Part print with two shaded views. Sizes in mm from the minimum x, y, z corner. A direction names the side the tool comes from. Round coordinates to 2 decimals unless told otherwise and drop trailing zeros. Order: outer loops, then holes, each group sorted by start corner. A loop starts at its lowest first (then second) coordinate and runs counter-clockwise, first axis right, second up. Notation, with made-up numbers: M 0,35 L 41,35 A28 ccw 41,71 Z; hole C -39,71.25 d11. An arc over 180 degrees is marked long. Put each result on its own line as item: value.
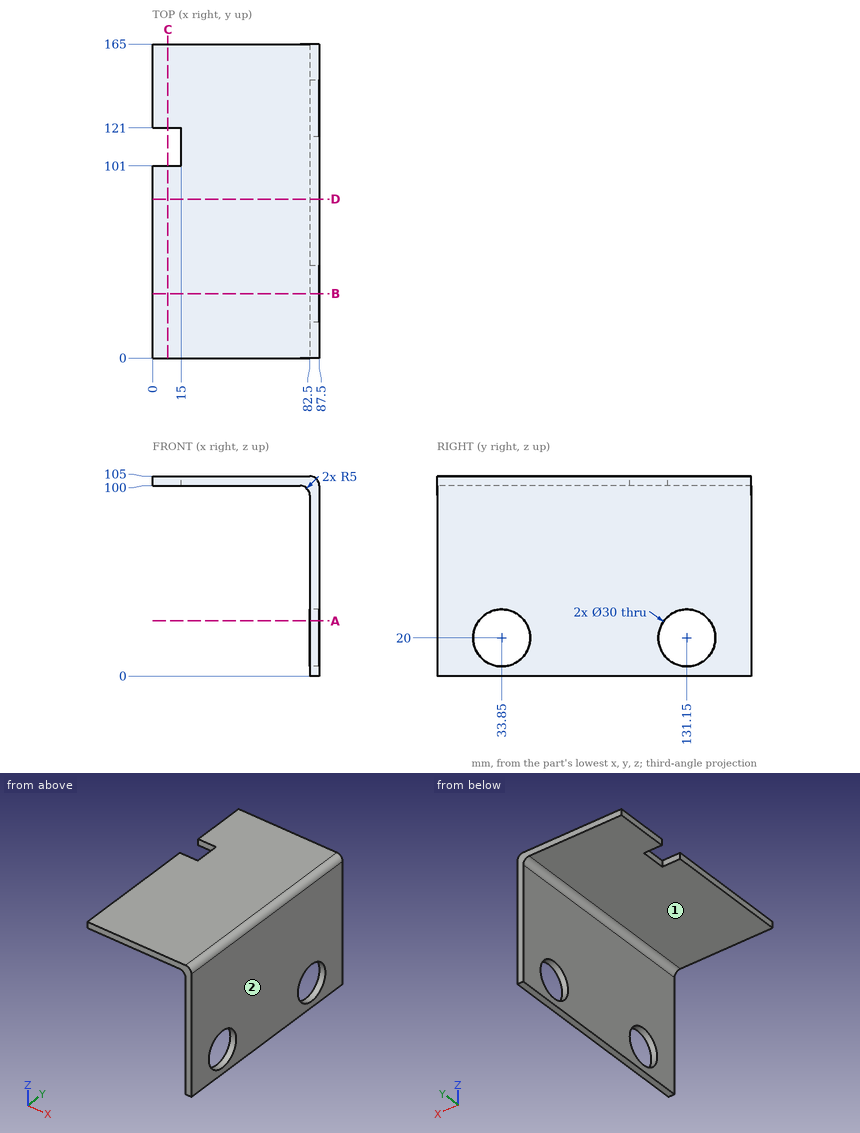
Item 1: Probe line 1 along Y through (x, z) = (83.65, 20); line 2 along Z through (x, y) = (83, 131); line 3 along X through (y, z) = (26.5, 64.5). List the from-to ranges inside material, lowest first. Write a range as [from, to].
Answers below:
line 1: [0, 18.85], [48.85, 116.15], [146.15, 165]
line 2: [0, 5], [35, 104.97]
line 3: [82.5, 87.5]
Item 2: Band-saw the part on C-C on x = 8. Give the cut face in (y, z).
Answers below:
outline: M 0,100 L 101,100 L 101,105 L 0,105 Z; M 121,100 L 165,100 L 165,105 L 121,105 Z
Item 3: Tool access for the marked faces 1 and 2: list every direction of +Z, -Z, +X, -X, +Y, -Y with a clear straight run to the whole face (end or side of a thin tool).
Answers below:
face 1: -Z, -X, +Y, -Y
face 2: +Z, -Z, +X, +Y, -Y
Item 4: Pin check, flat tips, straight feed: P1, Ø6, axis at x = 38.5, y = 40.5, coming from the -Z side; P2, Ø4, axis at y = 116, z = 102, coming from the -X side; P3, Ø4, axis at y = 49, z = 87, coming from the -X side. Stop position of each tip, or through.
Answers below:
P1: z = 100
P2: x = 15
P3: x = 82.5
Item 5: Band-saw the part on D-D on y = 83.5. Give the cut face in (x, z), and give its area (4 significant figures).
Answers below:
outline: M 0,100 L 77.5,100 A5 cw 82.5,95 L 82.5,0 L 87.5,0 L 87.5,100 A5 ccw 82.5,105 L 0,105 Z
area: 937.5 mm²
Item 6: Band-saw the part on B-B on y = 33.85. Give the cut face in (x, z).
Answers below:
outline: M 0,100 L 77.5,100 A5 cw 82.5,95 L 82.5,35 L 87.5,35 L 87.5,100 A5 ccw 82.5,105 L 0,105 Z; M 82.5,0 L 87.5,0 L 87.5,5 L 82.5,5 Z
Item 7: Band-saw the part on A-A on z = 29. Give the cut face in (x, y), and give its area (3 significant figures).
Answers below:
outline: M 82.5,0 L 87.5,0 L 87.5,21.85 L 82.5,21.85 Z; M 82.5,45.85 L 87.5,45.85 L 87.5,119.15 L 82.5,119.15 Z; M 82.5,143.15 L 87.5,143.15 L 87.5,165 L 82.5,165 Z
area: 585 mm²
